Here's how the part is built. I have some questions about the finished solid (model axes, mm). Round coordinates to 2 decimals unless told otherwise and drop trailing zeros. Write each loop counter-clockwise with the first axis right and the second up, starting at its lowest first coordinate (ties: lowest second). Pieces come first, ordered by that corner, then holes. Notation, with made-up numbers: M 36.5,-22.5 L 47.5,-22.5 A31 cw 47.5,14.5 Z; hole C 68,37 d5. An arc over 180 degrees is marked long. Write item = value, one per line. Start each with the question number.
(1) I want a section at A-A (y = 9). List the corners of the cut face in (x, z) for me.
(2) I want a section at D-D (x = -66). List the corners of the cut face in (y, z) for me, and give its area (3 significant figures).
(3) I need wall thicknesses on line 1 along Y through (x, z) = (-27, 1.5); line 2 along Y through (x, z) = (-44, 2.2); line 3 along Y through (x, z) = (-41.5, 0.1). Which ranges of each line are inside material? Lowest first, please.
(4) Will this pin go through, and if not, where does the flat tip stop? pin 1 Ø5 at (x, y) = (-46.5, -6.5) entering from -Z.
(5) I want a section at C-C (z = 0.65). List the corners of the cut face in (x, y) for me.
(6) I want a section at B-B (x = -43). List the corners of the cut face in (y, z) for me.
```python
from build123d import *

# Parameters (mm, degrees)
CROQUIS1_R              = 31.5
CROQUIS1_R_2            = 1.5
SALIENTE_EXTRUIR1_DEPTH = 3
CROQUIS4_R              = 2.5
CORTAR_EXTRUIR3_DEPTH   = 3


with BuildPart() as part:
    # Croquis1 → Saliente-Extruir1 (new body)
    with BuildSketch(Plane.XY):
        with Locations((-43.449193048, 8.207110309)):
            Circle(CROQUIS1_R)
        with Locations((-60.066202406, 24.824119667)):
            Circle(CROQUIS1_R_2, mode=Mode.SUBTRACT)
        with Locations((-26.83218369, 24.824119667)):
            Circle(CROQUIS1_R_2, mode=Mode.SUBTRACT)
        with Locations((-26.83218369, -8.409899049)):
            Circle(CROQUIS1_R_2, mode=Mode.SUBTRACT)
        with Locations((-60.066202406, -8.409899049)):
            Circle(CROQUIS1_R_2, mode=Mode.SUBTRACT)
    extrude(amount=SALIENTE_EXTRUIR1_DEPTH)

    # Croquis4 → Cortar-Extruir3 (cut)
    with BuildSketch(Plane(origin=(0, 0, 0), x_dir=(-1, 0, 0), z_dir=(0, 0, -1))):
        with Locations((43.449193048, 8.207110309)):
            Circle(CROQUIS4_R)
    extrude(amount=-CORTAR_EXTRUIR3_DEPTH, mode=Mode.SUBTRACT)


solid = part.part
```
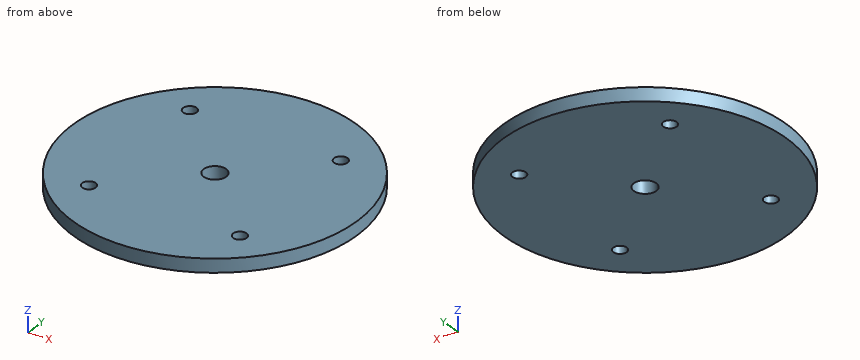
Returned:
q1.outline = M -74.94,0 L -45.82,0 L -45.82,3 L -74.94,3 Z; M -41.08,0 L -11.96,0 L -11.96,3 L -41.08,3 Z
q2.outline = M -13.79,0 L 30.2,0 L 30.2,3 L -13.79,3 Z
q2.area = 132 mm²
q3.line_1 = -18.66 to -9.9, -6.92 to 23.33, 26.31 to 35.07
q3.line_2 = -23.29 to 5.77, 10.65 to 39.7
q3.line_3 = -23.23 to 6.64, 9.77 to 39.65
q4.pin_1 = 0
q5.outline = C -43.45,8.21 d63; hole C -60.07,-8.41 d3; hole C -60.07,24.82 d3; hole C -43.45,8.21 d5; hole C -26.83,-8.41 d3; hole C -26.83,24.82 d3
q6.outline = M -23.29,0 L 5.75,0 L 5.75,3 L -23.29,3 Z; M 10.67,0 L 39.7,0 L 39.7,3 L 10.67,3 Z
